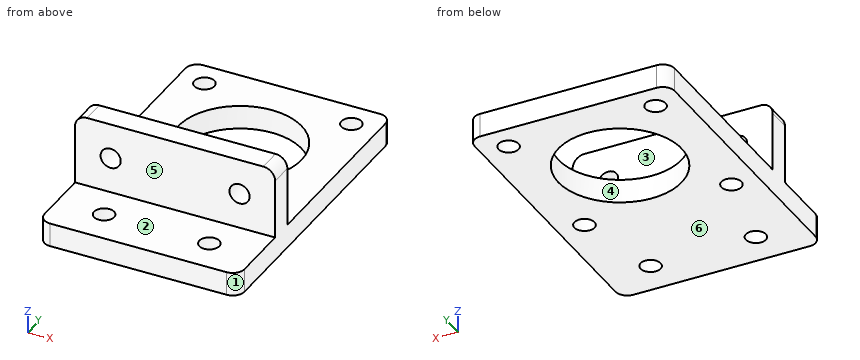
```python
from build123d import *

# Parameters (mm, degrees)
F0_R     = 2.125
F0_R_2   = 2.12
F0_R_3   = 13
F1_DEPTH = 5
F2_W     = 42.2
F2_H     = 5
F3_DEPTH = 15
F4_R     = 2.125
F5_DEPTH = 47.601
F6_R     = 2.5


with BuildPart() as f1:
    # F0 (on Top) → F1 (new body)
    with BuildSketch(Plane.XY):
        with BuildLine():
            Line((18.6, 21.1), (0, 21.1))
            Line((0, 21.1), (-18.6, 21.1))
            ThreePointArc((-18.6, 21.1), (-20.367767, 20.367767), (-21.1, 18.6))
            Line((-21.1, 18.6), (-21.1, -39))
            ThreePointArc((-21.1, -39), (-20.367767, -40.767767), (-18.6, -41.5))
            Line((-18.6, -41.5), (0, -41.5))
            Line((0, -41.5), (18.6, -41.5))
            ThreePointArc((18.6, -41.5), (20.367767, -40.767767), (21.1, -39))
            Line((21.1, -39), (21.1, 18.6))
            ThreePointArc((21.1, 18.6), (20.367767, 20.367767), (18.6, 21.1))
        make_face()
        with Locations((-11.1, -34)):
            Circle(F0_R, mode=Mode.SUBTRACT)
        with Locations((-15.5, -15.5)):
            Circle(F0_R_2, mode=Mode.SUBTRACT)
        with Locations((11.1, -34)):
            Circle(F0_R, mode=Mode.SUBTRACT)
        with Locations((15.5, -15.5)):
            Circle(F0_R, mode=Mode.SUBTRACT)
        with Locations((-15.5, 15.5)):
            Circle(F0_R, mode=Mode.SUBTRACT)
        Circle(F0_R_3, mode=Mode.SUBTRACT)
        with Locations((15.5, 15.5)):
            Circle(F0_R, mode=Mode.SUBTRACT)
    extrude(amount=F1_DEPTH)

    # F2 (on face) → F3 (join)
    with BuildSketch(Plane.XY.offset(5)):
        with Locations((0, -24)):
            Rectangle(F2_W, F2_H)
    extrude(amount=F3_DEPTH)

    # F4 (on face) → F5 (cut, through all)
    with BuildSketch(Plane.XZ.offset(26.5)):
        with Locations((-13.6, 12.5)):
            Circle(F4_R)
        with Locations((13.6, 12.5)):
            Circle(F4_R)
    extrude(amount=-F5_DEPTH, mode=Mode.SUBTRACT)

    # F6
    f6_edges = [f1.edges().sort_by_distance(p)[0] for p in [
        (-21.1, -24, 20),
        (21.1, -24, 20),
    ]]
    fillet(f6_edges, radius=F6_R)


solid = f1.part
```
Source: CAD feature listing. Evaluate the final solid. Frame: model axes, mm. Face numbers are marked on the shaded views. A direction names the side the tool comes from. Round coordinates to 2 decimals unless told otherwise and drop trailing zeros. Loops run counter-clockwise (first coordinate to the right, second up) from the corner with the lowest first, then second, coordinate; pieces in that order, holes last.
1. Ray query, L1, parallel to Y at x = -15.5, z = 1.6 (3 decimals); L2, parallel to Y at x = 11.1, z = 2.55 (3 decimals); L3, parallel to Z at x = 14.5, y = 13. Return the intervals inside material, ascending.
2. Access query for the marked faces 1, 2 and 3. Directions: +Z, -Z, +X, -X, +Y, -Y. A direction counts if a zero-diameter tool reaches every point of the face in a straight line with its end or side. Return the directions, or none.
3. Section query A-A on x = 0. Output: boundary loops of the cut face in (y, z).
4. Section query B-B on y = -15.5. Output: boundary loops of the cut face in (x, z) (3 decimals), and give its area (3 significant figures).
5. Contact query for flat-ended pins moving along their axis: pin 1 (5.5 mm diameter, centred on x = -11.1, y = -34, fed in from +Z); pin 2 (12 mm diameter, centred on x = -0.5, z = 9, fed in from +Y); pin 3 (4.5 mm diameter, centred on x = 1.5, z = 10.5, fed in from -Y); pin 4 (1.5 mm diameter, centred on x = 14.5, z = 6.5, fed in from +Y). Output: stop coordinate, or through.
6. Section query D-D on x = -15. Output: boundary loops of the cut face in (y, z).
7. Mould query, pull axis Y, two halves, no side actions, for the marked faces 4, 5 and 6. Classes: released by +Y, released by -Y, zero draft, split by the parting line, or undercut.
8. Section query C-C on z = 12.5. Output: boundary loops of the cut face in (x, y) (3 decimals), and give its area (4 significant figures).
Answers below:
1. L1: y = -41.5 to -17.62, -13.38 to 13.375, 17.625 to 21.1
1. L2: y = -41.5 to -36.125, -31.875 to -6.767, 6.767 to 21.1
1. L3: z = 0 to 5
2. face 1: +Z, -Z, +X, -Y
2. face 2: +Z, +X, -X, -Y
2. face 3: +Z, +X, -X, +Y
3. outline: (-41.5, 0) - (-13, 0) - (-13, 5) - (-21.5, 5) - (-21.5, 20) - (-26.5, 20) - (-26.5, 5) - (-41.5, 5) - close; (13, 0) - (21.1, 0) - (21.1, 5) - (13, 5) - close
4. outline: (-21.1, 0) - (-17.62, 0) - (-17.62, 5) - (-21.1, 5) - close; (-13.38, 0) - (13.375, 0) - (13.375, 5) - (-13.38, 5) - close; (17.625, 0) - (21.1, 0) - (21.1, 5) - (17.625, 5) - close
4. area: 169 mm2
5. pin 1: stops at z = 5
5. pin 2: stops at y = 21.1
5. pin 3: stops at y = -26.5
5. pin 4: stops at y = -21.5
6. outline: (-41.5, 0) - (-17.56, 0) - (-17.56, 5) - (-21.5, 5) - (-21.5, 10.9) - (-26.5, 10.9) - (-26.5, 5) - (-41.5, 5) - close; (-26.5, 14.1) - (-21.5, 14.1) - (-21.5, 20) - (-26.5, 20) - close; (-13.44, 0) - (13.43, 0) - (13.43, 5) - (-13.44, 5) - close; (17.57, 0) - (21.1, 0) - (21.1, 5) - (17.57, 5) - close
7. face 4: undercut
7. face 5: released by -Y
7. face 6: zero draft
8. outline: (-21.1, -26.5) - (-15.725, -26.5) - (-15.725, -21.5) - (-21.1, -21.5) - close; (-11.475, -26.5) - (11.475, -26.5) - (11.475, -21.5) - (-11.475, -21.5) - close; (15.725, -26.5) - (21.1, -26.5) - (21.1, -21.5) - (15.725, -21.5) - close
8. area: 168.5 mm2
